Geometry: final body of the model. Coordinates: model frame, mm. Round coordinates to 2 decimals unless told otherwise and drop trailing zeros. Write each loop counter-clockwise with the first axis right and the second up, starting at its lowest first coordinate (ties: lowest second). Pieces come first, ordered by that corner, then holes. Notation, with made-up numbers: M 51,16.25 L 100,16.25 A20 ccw 100,35.25 Z; hole C -26,74 d9. An arc over 180 degrees is marked long. Use one line per item in the form item = value. Start each with the question number.
Autodesk Inventor part; units mm, degrees
ref_plane "YZ Plane" through (0, 0, 0) normal (1, 0, 0) x (0, 1, 0)
ref_plane "XZ Plane" through (0, 0, 0) normal (0, 1, 0) x (-1, 0, 0)
ref_plane "XY Plane" through (0, 0, 0) normal (0, 0, 1) x (1, 0, 0)
sketch "Sketch1" plane through (0, 0, 0) normal (0, 1, 0) x (-1, 0, 0)
  circle A0 centre (0, 0) radius 1.27
  line L0 (0, 1.27) -> (0, 4.98) construction
  line L1 (0, 4.98) -> (0, -17.37) construction
  line L2 (0, -6.195) -> (6.075, -6.195) construction
  line L3 (0, 4.98) -> (0.075, 4.98)
  line L4 (6.075, -1.02) -> (6.075, -6.195)
  line L5 (0, 4.98) -> (-0.075, 4.98)
  line L6 (-6.075, -1.02) -> (-6.075, -6.195)
  line L7 (-6.075, -6.195) -> (0, -6.195) construction
  arc A1 (6.075, -1.02) -> (0.075, 4.98) centre (0.075, -1.02) ccw
  arc A2 (-0.075, 4.98) -> (-6.075, -1.02) centre (-0.075, -1.02) ccw
  circle A3 centre (0, -12.39) radius 1.27
  line L8 (0, -13.66) -> (0, -17.37) construction
  line L9 (0, -17.37) -> (0, 4.98) construction
  line L10 (0, -17.37) -> (0.075, -17.37)
  line L11 (0, -17.37) -> (-0.075, -17.37)
  arc A4 (0.075, -17.37) -> (6.075, -11.37) centre (0.075, -11.37) ccw
  arc A5 (-6.075, -11.37) -> (-0.075, -17.37) centre (-0.075, -11.37) ccw
  line L12 (6.075, -11.37) -> (6.075, -6.195)
  line L13 (-6.075, -11.37) -> (-6.075, -6.195)
  point P0 (-6.075, 4.98)
  point P1 (-6.075, -17.37)
  point P2 (6.075, -3.6075)
  dimension "d0" = 2.54
  dimension "d1" = 3.71
  dimension "d2" = 22.35
  dimension "d3" = 6.075
  dimension "d4" = 6.075
  dimension "d5" = 6
  dimension "d6" = 6
  dimension "d7" = 12.15
extrude "Extrusion1" add sketch "Sketch1" along normal blind 1.9
fillet "Fillet1" radius 1.5 8 edges at (6.075, 1.9, -3.6075) (4.3176, 1.9, -15.6126) (-0.0375, 1.9, -17.37) (-4.3176, 1.9, -15.6126) (-6.075, 1.9, -3.6075) (-4.3176, 1.9, 3.2226) (-0.0375, 1.9, 4.98) (4.3176, 1.9, 3.2226)
1. Pull-direction query (Z, two-part tool) for faces 1 (the face through (4.36, 0.2, 3.18)), 2 (the face through (-5.624, 1.472, -6.123)), 3 (the face through (-1.2, 0.9, -12.8)); classes: released by +Z, released by -Z, zero draft, split by the parting line, or undercut.
2. Ray query, probe 1 along Z at (x, y) = (0, 0.4); probe 2 along Z at (x, y) = (-0.5, 1.7); probe 3 along X at (y, z) = (0.75, -0.5). Return the intervals inside material, ascending.
3. Section query A-A (z = -9.25). Return loops of the section in (x, y) (3 decimals).
4. Section query B-B (y = 1.5). Return loops of the section in (x, z) (3 decimals).
Checks:
q1.face_1 = released by +Z
q1.face_2 = zero draft
q1.face_3 = undercut
q2.probe_1 = -17.37 to -13.66, -11.12 to -1.27, 1.27 to 4.98
q2.probe_2 = -16.6 to -13.56, -11.22 to -1.17, 1.17 to 4.21
q2.probe_3 = -6.01 to -1.17, 1.17 to 6.01
q3.outline = M -6.075,0 L 6.075,0 L 6.075,0.4 A1.5 ccw 4.575,1.9 L -4.575,1.9 A1.5 ccw -6.075,0.4 Z
q4.outline = M -5.595,-11.37 A5.52 ccw -0.075,-16.89 L 0.075,-16.89 A5.52 ccw 5.595,-11.37 L 5.595,-1.02 A5.52 ccw 0.075,4.5 L -0.075,4.5 A5.52 ccw -5.595,-1.02 Z; hole C 0,-12.39 d2.54; hole C 0,0 d2.54
